Autodesk Inventor part; units mm, degrees
ref_plane "YZ Plane" through (0, 0, 0) normal (1, 0, 0) x (0, 1, 0)
ref_plane "XZ Plane" through (0, 0, 0) normal (0, 1, 0) x (-1, 0, 0)
ref_plane "XY Plane" through (0, 0, 0) normal (0, 0, 1) x (1, 0, 0)
sketch "Sketch1" plane through (0, 0, 0) normal (1, 0, 0) x (0, 1, 0)
  line L0 (2, 5) -> (9, 5)
  line L1 (9, 5) -> (9, 3)
  line L2 (9, 3) -> (10, 3)
  line L3 (10, 3) -> (10, 10)
  line L4 (10, 10) -> (8, 10)
  line L5 (8, 10) -> (8, 50)
  line L6 (8, 50) -> (10, 50)
  line L7 (10, 50) -> (10, 75)
  line L8 (10, 75) -> (0, 75)
  line L9 (0, 75) -> (0, 50)
  line L10 (0, 50) -> (2, 50)
  line L11 (2, 50) -> (2, 5)
  line L12 (24.985, 0) -> (-21.0801, 0)
  line L13 (0, 63.0325) -> (0, -71.2298) construction
  point P0 (0, 0)
  point P1 (5.5, 5)
  point P2 (5, 75)
  dimension "d0" = 150
  dimension "d1" = 10
  dimension "d2" = 2
  dimension "d3" = 7
  dimension "d4" = 1
  dimension "d5" = 7
  dimension "d6" = 2
  dimension "d7" = 25
  dimension "d8" = 47
  dimension "d9" = 0
  dimension "d10" = 70
revolve "Revolution1" add sketch "Sketch1" angle 360 about axis through (0, 24.985, 0) along (0, -1, 0)
sketch "Sketch2" plane through (0, 2, 0) normal (0, -1, 0) x (1, 0, 0)
  point P0 (0, 0)
sketch "Sketch3" plane through (0, 0, 0) normal (0, -1, 0) x (1, 0, 0)
  circle A0 centre (0, 0) radius 62.5
  circle A1 centre (62.5, 0) radius 4
  dimension "d12" = 125
  dimension "d13" = 8
hole "Hole1" at (62.5, 0, 0) direction (0, 1, 0) diameter 8 end through all
chamfer "Chamfer1" distance 0.5 angle 45 1 edges at (62.5, 10, 4)
pattern_circular "Circular Pattern1" count 6 over 360 about axis through (0, 5, 0) along (0, -1, 0) of "Hole1"
properties part number "10_Nap_cua_tham"
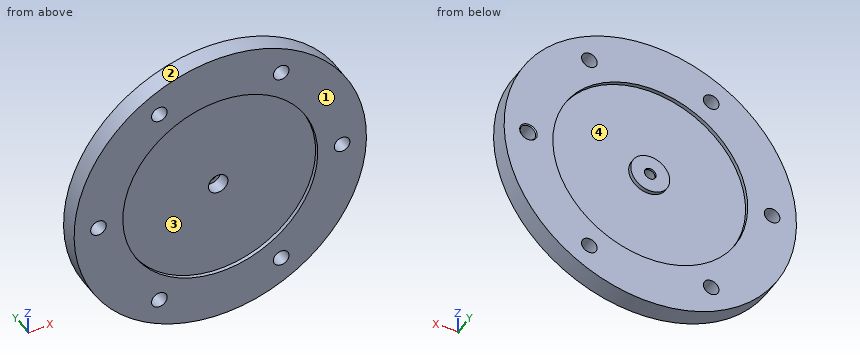
The listing builds one solid part. Answer for the finished solid, in the listing's coordinates (mm). Face numbers are marked on the shaded views. Round coordinates to 2 decimals unless told otherwise and drop trailing zeros. Write each loop counter-clockwise with the first axis right and the second up, starting at its lowest first coordinate (ties: lowest second). Pieces come first, ordered by that corner, then holes. Notation, with made-up numbers: (82, 88.5) - (99, 88.5) arc R20 cw to (99, 108.5) - close; hole circle Ø10 at (-14.75, -4). An arc over 180 degrees is marked (long way). Use one line per item in the form item = value. Start each with the question number.
Item 1: A cutting plane is placed at B-B (z = 0). Give the number of separate pieces and of enclosed holes in the cut face, plus the area to 3 significant figures.
Item 2: A cutting plane is placed at C-C (x = 30). Write down the section's boundary in (y, z).
Item 3: A cutting plane is placed at D-D (z = 46). Write down the section's boundary in (x, y), plus the area to 3 significant figures.
Item 4: A cutting plane is placed at A-A (x = 0). Write down the section's boundary in (y, z).
Item 5: Flat-ended cylindrical pins translate along their axes: pin 1 Ø4 at (y, z) = (6.5, -5) entering from -X; pin 2 Ø10.5 at (x, z) = (62.5, 0) entering from +Y; pin 3 Ø3 at (y, z) = (7, -13.5) entering from -X; pin 4 Ø2 at (x, y) = (-15, 3.5) entering from -Z. Find the tip coordinate at first contact, or state that the pin passes through.
Item 6: Find the intervals of material crossed by line 1 (X direction, y = 6.75, z = 0); line 2 (X direction, y = 1, z = 0); line 3 (Z direction, x = 0, y = 9.5), in increasing order. Write a range as [from, to].
Item 7: Determine the mould class of the marked faces 1, 2, 3 and 4 for opening direction Z: +Z half, -Z half, draft (parallel to the pull), parting line (faces both ways), or undercut.
The answers:
q1.separate_pieces = 4
q1.enclosed_holes = 0
q1.area = 904 mm^2
q2.outline = (0, -68.74) - (10, -68.74) - (10, -57.93) - (0, -57.93) - close; (0, -50.33) - (10, -50.33) - (10, -40) - (8, -40) - (8, 40) - (10, 40) - (10, 50.33) - (0, 50.33) - (0, 40) - (2, 40) - (2, -40) - (0, -40) - close; (0, 57.93) - (10, 57.93) - (10, 68.74) - (0, 68.74) - close
q3.outline = (-59.24, 0) - (-19.6, 0) - (-19.6, 2) - (19.6, 2) - (19.6, 0) - (59.24, 0) - (59.24, 10) - (19.6, 10) - (19.6, 8) - (-19.6, 8) - (-19.6, 10) - (-59.24, 10) - close
q3.area = 1,030 mm^2
q4.outline = (0, -75) - (10, -75) - (10, -50) - (8, -50) - (8, -10) - (10, -10) - (10, -3) - (9, -3) - (9, -5) - (2, -5) - (2, -50) - (0, -50) - close; (0, 50) - (2, 50) - (2, 5) - (9, 5) - (9, 3) - (10, 3) - (10, 10) - (8, 10) - (8, 50) - (10, 50) - (10, 75) - (0, 75) - close
q5.pin_1 = -74.94
q5.pin_2 = 10
q5.pin_3 = -74.03
q5.pin_4 = -73.68
q6.line_1 = [-75, -66.5], [-58.5, -5], [5, 58.5], [66.5, 75]
q6.line_2 = [-75, -66.5], [-58.5, -50], [50, 58.5], [66.5, 75]
q6.line_3 = [-75, -50], [-10, -3], [3, 10], [50, 75]
q7.face_1 = draft
q7.face_2 = parting line
q7.face_3 = undercut
q7.face_4 = undercut
